Design review of the part built by this model. Coordinates are the model's own, in mm. Face numbers are marked on the shaded views. A direction names the side the tool comes from. Give positions to 0.01 mm unless a question says otherwise; leave off trailing zeros. Loops run counter-clockwise (first coordinate to the right, second up) from the corner with the lowest first, then second, coordinate; pieces in that order, holes last. Notation, with made-up numbers: (76, -35.75) -> (124, -35.75) arc R18 ccw to (124, -20.75) -> close; hole circle Ø10 at (79, 80). An arc over 180 degrees is marked (long way). Answer as CSV lines item,"result".
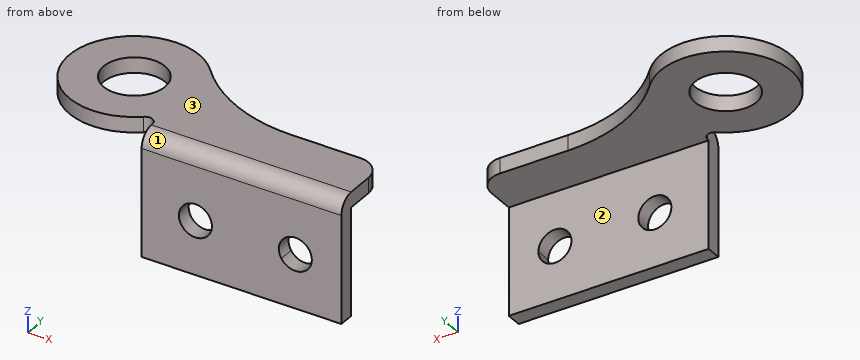
from build123d import *

# Parameters (mm, degrees)
EXTRUDE_1_DEPTH = 2
SKETCH_2_W      = 26
SKETCH_2_H      = 16
SKETCH_2_R      = 2.15
EXTRUDE_2_DEPTH = 2
FILLET_1_R      = 2


with BuildPart() as part:
    # 草图1 → 凸台-拉伸1 (new body)
    with BuildSketch(Plane.XY):
        with BuildLine():
            ThreePointArc((-5.068859013, 5.89218325), (1.666665094, 0.98511468), (9.817268595, -0.751050494))
            Line((9.817268595, -0.751050494), (18.641752073, -0.751050494))
            ThreePointArc((18.641752073, -0.751050494), (20.763072416, -1.62973015), (21.641752073, -3.751050494))
            Line((21.641752073, -3.751050494), (21.641752073, -7.251050494))
            Line((21.641752073, -7.251050494), (-4.358247927, -7.251050494))
            Line((-4.358247927, -7.251050494), (-4.358247927, -7.051906608))
            ThreePointArc((-4.358247927, -7.051906608), (-4.931001298, -6.147771487), (-5.993168562, -6.279329241))
            ThreePointArc((-5.993168562, -6.279329241), (-19.783987468, 0.888803553), (-5.068859013, 5.89218325))
        make_face()
        with BuildLine():
            ThreePointArc((-11.358247927, -3.751050494), (-7.358247927, 0.248949506), (-11.358247927, 4.248949506))
            ThreePointArc((-11.358247927, 4.248949506), (-15.358247927, 0.248949506), (-11.358247927, -3.751050494))
        make_face(mode=Mode.SUBTRACT)
        Polygon((19.641752073, -9.251050494), (-2.358247927, -9.251050494), (-4.358247927, -9.251050494), (-4.358247927, -7.251050494), (21.641752073, -7.251050494), (21.641752073, -9.251050494), align=None)
    extrude(amount=EXTRUDE_1_DEPTH)

    # 草图2 → 凸台-拉伸2 (add)
    with BuildSketch(Plane.XZ.offset(9.251050494)):
        with Locations((8.641752073, -6)):
            Rectangle(SKETCH_2_W, SKETCH_2_H)
        with Locations((2.641752073, -7)):
            Circle(SKETCH_2_R, mode=Mode.SUBTRACT)
        with BuildLine():
            ThreePointArc((13.82437189, -8.148751179), (15.043783592, -4.93482841), (17.791752073, -7))
            ThreePointArc((17.791752073, -7), (16.239720553, -9.06517159), (13.82437189, -8.148751179))
        make_face(mode=Mode.SUBTRACT)
    extrude(amount=-EXTRUDE_2_DEPTH)

    # 圆角1
    fillet_1_edges = [part.edges().sort_by_distance(p)[0] for p in [
        (8.641752073, -9.251050494, 2),
    ]]
    fillet(fillet_1_edges, radius=FILLET_1_R)


solid = part.part
Q1. We need section B-B, the plane y = -1.25. State the section outline as (x, z) points, and give its area (3 significant figures).
Filled sheet:
outline,"(-19.67, 0) -> (-15.07, 0) -> (-15.07, 2) -> (-19.67, 2) -> close; (-7.65, 0) -> (20.3, 0) -> (20.3, 2) -> (-7.65, 2) -> close"
area,"65.1 mm^2"
Q2. Clearance check with flat-ended pins moving along their axes: pin 1 Ø0.7 at (y, z) = (-8.5, -5.5) entering from -X; pin 2 Ø4 at (x, z) = (6.5, -5) entering from +Y; pin 3 Ø2 at (x, z) = (14.5, 0.5) entering from +Y. State where each tip first meets the part, or that it passes through.
Filled sheet:
pin 1,"stops at x = -4.36"
pin 2,"stops at y = -7.25"
pin 3,"stops at y = -0.75"
Q3. We need section D-D, the plane x = -16. State the section outline as (y, z) points.
Filled sheet:
outline,"(-6.81, 0) -> (7.31, 0) -> (7.31, 2) -> (-6.81, 2) -> close"
Q4. We need section A-A, the plane z = -6.25. State the section outline as (x, y) points.
Filled sheet:
outline,"(-4.36, -9.25) -> (0.63, -9.25) -> (0.63, -7.25) -> (-4.36, -7.25) -> close; (4.66, -9.25) -> (13.63, -9.25) -> (13.63, -7.25) -> (4.66, -7.25) -> close; (17.66, -9.25) -> (21.64, -9.25) -> (21.64, -7.25) -> (17.66, -7.25) -> close"
Q5. We need section C-C, the plane z = -10.5. State the section outline as (x, y) points.
Filled sheet:
outline,"(-4.36, -9.25) -> (21.64, -9.25) -> (21.64, -7.25) -> (-4.36, -7.25) -> close"
Q6. To check wall thickness, follow probe 1 along Z at (x, y) = (8, -5.25); probe 2 along X at (y, z) = (3, 0.5); probe 3 along Y at (x, z) = (-2.5, -2.25). State the ranges of each line that lie inside material, in increasing order. Write a range as from..to.
Filled sheet:
probe 1,"z = 0..2"
probe 2,"x = -19.35..-14.26, -8.45..-1.84"
probe 3,"y = -9.25..-7.25"
Q7. For the marked faces 1, 2 and 3, list the 3-axis set-ups (+Z, -Z, +X, -X, +Y, -Y) from which the entire face can be reached by the end or side of a thin tool; tool diameter is ignored.
Filled sheet:
face 1,"+Z, +X, -Y"
face 2,"-Z, +X, -X, +Y"
face 3,"+Z, +X, -X, +Y, -Y"
